Source: CAD feature listing. Evaluate the final solid. Frame: model axes, mm. Coordinates: 2 decimals unless noted, no trailing zeros. Write each loop counter-clockwise with the first axis right and the second up, starting at its lowest first coordinate (ties: lowest second). Pieces come first, ordered by that corner, then holes. Notation, with made-up numbers: (5, -3.75) - (15, -3.75) arc R28 ccw to (15, 34.25) - close; hole circle Ø8 at (-25, 12.25). An arc over 180 degrees is marked (long way). One line per question, with ' | ' between items. Start each with the question number.
Q1. Cut plane A-A, the plane z = 3.25. Return loops of the section in (x, y).
Q2. Draft query along X for faces 1 (the face through (-78.21, 2.54, 3.01)), 2 (the face through (-48.128, 2.535, 2.844)), 3 (the face through (1, 5, 3)). Return one class per face: +X half, -X half, draft (parallel to the pull), parting line (faces both ways), or undercut.
Q3. Contact query for flat-ended pins moving along their axis: P1, Ø3, axis at x = -45.69, z = 3.39, coming from the +Y side (3 decimals); P2, Ø3, axis at y = 2.5, z = 1.5, coming from the +X side. Output: stop coordinate, or through.
Q4. Line query: line 1 (X direction, y = 3.7, z = 1.75); line 2 (X direction, y = 3.4, z = 4.75); line 3 (Z direction, x = 73, y = 3.2). Output: solid intervals per line, ascending.
Q5. Cut plane B-B, the plane y = 2.3. Return loops of the section in (x, z), plus the area to 3 significant figures.
Q6. Cut plane C-C, the plane x = 52.5. Return loops of the section in (y, z).
```python
from build123d import *

# Parameters (mm, degrees)
BOSS_EXTRUDE1_DEPTH = 5
CUT_EXTRUDE1_REACH  = 88.258
SKETCH3_R           = 2.5


with BuildPart() as part:
    # Sketch2 → Boss-Extrude1 (new body)
    with BuildSketch(Plane(origin=(0, 0, 0), x_dir=(1, 0, 0), z_dir=(0, 1, 0))):
        with BuildLine():
            Line((-80.680626491, 1.660466244), (79.319373509, 1.44949578))
            ThreePointArc((79.319373509, 1.44949578), (84.312776341, -3.557092695), (79.306187867, -8.550495527))
            Line((79.306187867, -8.550495527), (-80.693812133, -8.339525063))
            ThreePointArc((-80.693812133, -8.339525063), (-85.687214966, -3.332936588), (-80.680626491, 1.660466244))
        make_face()
    extrude(amount=BOSS_EXTRUDE1_DEPTH)

    # Sketch3 → Cut-Extrude1 (cut, up to next)
    with BuildSketch(Plane(origin=(0, 5, 0), x_dir=(1, 0, 0), z_dir=(0, 1, 0)), mode=Mode.PRIVATE) as cut_extrude1_sk1:
        with Locations(Location((-80.687219312, -3.33952941, 0), (0, 0, 270))):
            Circle(SKETCH3_R)
    cut_extrude1_tool1 = extrude(cut_extrude1_sk1.sketch, amount=-CUT_EXTRUDE1_REACH, mode=Mode.PRIVATE) & part.part
    # Sketch3 → Cut-Extrude1 (cut, up to next)
    with BuildSketch(Plane(origin=(0, 5, 0), x_dir=(1, 0, 0), z_dir=(0, 1, 0)), mode=Mode.PRIVATE) as cut_extrude1_sk2:
        with Locations(Location((79.312780688, -3.550499874, 0), (0, 0, 270))):
            Circle(SKETCH3_R)
    cut_extrude1_tool2 = extrude(cut_extrude1_sk2.sketch, amount=-CUT_EXTRUDE1_REACH, mode=Mode.PRIVATE) & part.part
    # Sketch3 → Cut-Extrude1 (cut, up to next)
    with BuildSketch(Plane(origin=(0, 5, 0), x_dir=(1, 0, 0), z_dir=(0, 1, 0)), mode=Mode.PRIVATE) as cut_extrude1_sk3:
        with Locations(Location((-45.687249738, -3.385679158, 0), (0, 0, 270))):
            Circle(SKETCH3_R)
    cut_extrude1_tool3 = extrude(cut_extrude1_sk3.sketch, amount=-CUT_EXTRUDE1_REACH, mode=Mode.PRIVATE) & part.part
    add(cut_extrude1_tool1.solids().sort_by_distance((-80.687219, 5, 3.339529))[0], mode=Mode.SUBTRACT)
    add(cut_extrude1_tool2.solids().sort_by_distance((79.312781, 5, 3.5505))[0], mode=Mode.SUBTRACT)
    add(cut_extrude1_tool3.solids().sort_by_distance((-45.68725, 5, 3.385679))[0], mode=Mode.SUBTRACT)


solid = part.part
```
Reply:
1) outline: (-85.69, 0) - (-83.19, 0) - (-83.19, 5) - (-85.69, 5) - close; (-78.19, 0) - (-48.18, 0) - (-48.18, 5) - (-78.19, 5) - close; (-43.19, 0) - (76.83, 0) - (76.83, 5) - (-43.19, 5) - close; (81.79, 0) - (84.3, 0) - (84.3, 5) - (81.79, 5) - close
2) face 1: undercut | face 2: undercut | face 3: draft
3) P1: passes through | P2: stops at x = 84.28
4) line 1: x = -85.43 to -82.62, -78.76 to -47.58, -43.8 to 77.58, 81.05 to 83.98 | line 2: x = -85.48 to -82.75, -78.62 to -47.78, -43.59 to 77.12, 81.51 to 84.17 | line 3: z = -1.46 to 8.54
5) outline: (-80.69, 8.34) arc R5 ccw to (-80.68, -1.66) - (79.32, -1.45) arc R5 ccw to (79.31, 8.55) - close; hole circle Ø5 at (-80.69, 3.34); hole circle Ø5 at (-45.69, 3.39); hole circle Ø5 at (79.31, 3.55) | area: 1,620 mm^2
6) outline: (0, -1.48) - (5, -1.48) - (5, 8.52) - (0, 8.52) - close
